Part model, mm, in its own coordinate system. Face numbers are marked on the shaded views. A direction names the side the tool comes from. Round coordinates to 2 decimals unless told otherwise and drop trailing zeros. Order: outer loops, then holes, each group sorted by start corner. A loop starts at its lowest first (then second) coordinate and runs counter-clockwise, first axis right, second up. Notation, with made-up numbers: (81.25, 75) - (112.25, 75) arc R18 ccw to (112.25, 88) - close; hole circle Ø1 at (-38.75, 68). An arc over 180 degrees is marked (long way). Return JSON: item names as keys, results as strings. Group by question number.
Item 1: Two-plate mould, pull along Z, no slides. Class the marked faces 3, 4, 5 and 6: released by +Z, released by -Z, zero draft, split by the parting line, or undercut.
Item 2: Drop flat-ended pins along their axis: pin 1 (10 mm diameter, centred on x = 39.878, z = -12.7, fed in from +Y) (3 decimals); pin 2 (0.5 mm diameter, centred on x = 24.5, z = -27, fed in from -Y); pin 3 (1.6 mm diameter, centred on x = 10.5, z = -27.5, fed in from -Y). Give the stop position or say it passes through.
Item 3: Tool access for the marked faces 1 and 2: list every direction of +Z, -Z, +X, -X, +Y, -Y with a clear straight run to the whole face (end or side of a thin tool).
Item 4: Probe probe 1 along Z at (x, y) = (29.5, 21) (3 decimals); probe 2 along Y at (x, z) = (12, -27); probe 3 along X at (y, z) = (30, -26). List the from-to ranges inside material, lowest first.
Item 5: Saw through at C-C on y = 30.48. List the corners of the cut face in (x, z) (3 decimals), and give its area (3 significant figures).
Item 6: Saw through at D-D on z = -15. List the corners of the cut face in (x, y) (3 decimals), and give its area (3 significant figures).
Item 7: Saw through at B-B on x = 18.5. List the corners of the cut face in (y, z) (3 decimals), and give its area (3 significant figures).
Item 8: Saw through at A-A on x = 12.7. State how many separate pieces and enclosed holes the cut face has, and give its area (3 significant figures).
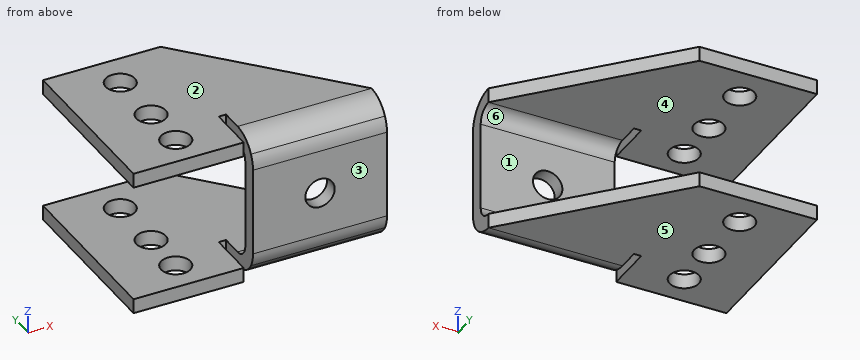
```python
from build123d import *

# Parameters (mm, degrees)
BOSS_EXTRUDE1_DEPTH     = 3.175
SKETCH2_W               = 28.956
SKETCH2_H               = 3.175
BOSS_EXTRUDE2_DEPTH     = 25.4
CUT_EXTRUDE1_DEPTH      = 74.581568589
CUT_EXTRUDE1_DEPTH_BACK = 74.581568589
SKETCH3_R               = 3.175
CUT_EXTRUDE2_DEPTH      = 71.646025975
CUT_EXTRUDE2_DEPTH_BACK = 71.646025975
SKETCH6_R               = 3.175
CUT_EXTRUDE3_DEPTH      = 74.581568589
CUT_EXTRUDE3_DEPTH_BACK = 74.581568589
SKETCH7_W               = 25.4
SKETCH7_H               = 0.79375
CONVERT_SOLID1_START    = 23.8125
CONVERT_SOLID1_DEPTH    = 30.5435
CONVERT_SOLID1_2_DEPTH  = 1.5875
CONVERT_SOLID1_START_2  = 25.4
CONVERT_SOLID1_3_DEPTH  = 28.956


# Read off the part's stored shape, not the designer's step: Convert-Solid1
with BuildPart() as part:
    # Sketch1 → Boss-Extrude1 (new body)
    with BuildSketch(Plane.XY):
        Polygon((54.356, 6.35), (25.4, 38.1), (0, 38.1), (0, 0), (54.356, 0), align=None)
    boss_extrude1 = extrude(amount=BOSS_EXTRUDE1_DEPTH)

    # Sketch2 → Boss-Extrude2 (add)
    with BuildSketch(Plane(origin=(0, 0, 0), x_dir=(-1, 0, 0), z_dir=(0, 0, -1))):
        with Locations((-39.878, 1.5875)):
            Rectangle(SKETCH2_W, SKETCH2_H)
    extrude(amount=BOSS_EXTRUDE2_DEPTH)

    # Mirror1: Boss-Extrude1 across plane
    add(boss_extrude1.mirror(Plane.XY.offset(-12.7)))

    # Sketch3 → Cut-Extrude1 (cut, two sides: drawn at the far end of the back side and taken through both)
    with BuildSketch(Plane.XY.offset(3.175).offset(-CUT_EXTRUDE1_DEPTH_BACK)):
        with Locations((12.7, 7.62)):
            Circle(SKETCH3_R)
        with Locations((12.7, 17.78)):
            Circle(SKETCH3_R)
        with Locations((12.7, 30.48)):
            Circle(SKETCH3_R)
    extrude(amount=CUT_EXTRUDE1_DEPTH + CUT_EXTRUDE1_DEPTH_BACK, mode=Mode.SUBTRACT)

    # Sketch6 → Cut-Extrude2 (cut, two sides: drawn at the far end of the back side and taken through both)
    with BuildSketch(Plane(origin=(0, 3.175, 0), x_dir=(1, 0, 0), z_dir=(0, 1, 0)).offset(-CUT_EXTRUDE2_DEPTH_BACK)):
        with Locations(Location((39.878, 12.7, 0), (0, 0, 270))):
            Circle(SKETCH6_R)
    extrude(amount=CUT_EXTRUDE2_DEPTH + CUT_EXTRUDE2_DEPTH_BACK, mode=Mode.SUBTRACT)

    # Sketch7 → Cut-Extrude3 (cut, two sides: drawn at the far end of the back side and taken through both)
    with BuildSketch(Plane(origin=(0, 0, -28.575), x_dir=(-1, 0, 0), z_dir=(0, 0, -1)).offset(-CUT_EXTRUDE3_DEPTH_BACK)):
        with Locations((-12.7, 0.396875)):
            Rectangle(SKETCH7_W, SKETCH7_H)
    extrude(amount=CUT_EXTRUDE3_DEPTH + CUT_EXTRUDE3_DEPTH_BACK, mode=Mode.SUBTRACT)

    # Convert-Solid1 outline → Convert-Solid1 (cut)
    with BuildSketch(Plane.YZ.offset(CONVERT_SOLID1_START)):
        with BuildLine():
            Line((0, -28.575), (6.35, -28.575))
            ThreePointArc((6.35, -28.575), (3.174999999, -27.724261314), (0.850738685, -25.4))
            ThreePointArc((0.850738685, -25.4), (0.216371003, -23.868500936), (0, -22.225))
            Line((0, -22.225), (0, -28.575))
        make_face()
        with BuildLine():
            Line((0, 3.175), (0, -3.175))
            ThreePointArc((0, -3.175), (0.216371003, -1.531499064), (0.850738685, 0))
            ThreePointArc((0.850738685, 0), (3.174999999, 2.324261314), (6.35, 3.175))
            Line((6.35, 3.175), (0, 3.175))
        make_face()
    extrude(amount=CONVERT_SOLID1_DEPTH, mode=Mode.SUBTRACT)

    # Convert-Solid1 2 outline → Convert-Solid1 2 (cut)
    with BuildSketch(Plane.YZ.offset(CONVERT_SOLID1_START)):
        with BuildLine():
            Line((6.35, -28.575), (11.1125, -28.575))
            Line((11.1125, -28.575), (11.1125, -25.4))
            Line((11.1125, -25.4), (0.850738685, -25.4))
            ThreePointArc((0.850738685, -25.4), (3.174999999, -27.724261314), (6.35, -28.575))
        make_face()
        with BuildLine():
            Line((0.850738685, 0), (11.1125, 0))
            Line((11.1125, 0), (11.1125, 3.175))
            Line((11.1125, 3.175), (6.35, 3.175))
            ThreePointArc((6.35, 3.175), (3.174999999, 2.324261314), (0.850738685, 0))
        make_face()
    extrude(amount=CONVERT_SOLID1_2_DEPTH, mode=Mode.SUBTRACT)

    # Convert-Solid1 3 outline → Convert-Solid1 3 (add)
    with BuildSketch(Plane.YZ.offset(CONVERT_SOLID1_START_2)):
        with BuildLine():
            Line((3.175, -25.4), (6.35, -25.4))
            ThreePointArc((6.35, -25.4), (4.10493597, -24.47006403), (3.175, -22.225))
            Line((3.175, -22.225), (3.175, -25.4))
        make_face()
        with BuildLine():
            Line((3.175, 0), (3.175, -3.175))
            ThreePointArc((3.175, -3.175), (4.10493597, -0.92993597), (6.35, 0))
            Line((6.35, 0), (3.175, 0))
        make_face()
    extrude(amount=CONVERT_SOLID1_3_DEPTH)


solid = part.part
```
Filled in:
{
 "1": {"face 3": "zero draft", "face 4": "undercut", "face 5": "released by -Z", "face 6": "undercut"},
 "2": {"pin 1": "stops at y = 3.175", "pin 2": "stops at y = 11.11", "pin 3": "stops at y = 0.79"},
 "3": {"face 1": "+X, -X, +Y", "face 2": "+Z, +X, -X, +Y, -Y"},
 "4": {"probe 1": "z = -28.575 to -25.4, 0 to 3.175", "probe 2": "y = 0.79 to 4.52, 10.72 to 14.68, 20.88 to 27.38, 33.58 to 38.1", "probe 3": "x = 0 to 9.56, 15.84 to 32.79"},
 "5": {"outline": "(0, -28.575) - (9.525, -28.575) - (9.525, -25.4) - (0, -25.4) - close; (0, 0) - (9.525, 0) - (9.525, 3.175) - (0, 3.175) - close; (15.875, -28.575) - (32.349, -28.575) - (32.349, -25.4) - (15.875, -25.4) - close; (15.875, 0) - (32.349, 0) - (32.349, 3.175) - (15.875, 3.175) - close", "area": "165 mm^2"},
 "6": {"outline": "(25.4, 0) - (37.689, 0) - (37.689, 3.175) - (25.4, 3.175) - close; (42.067, 0) - (54.356, 0) - (54.356, 3.175) - (42.067, 3.175) - close", "area": "78.0 mm^2"},
 "7": {"outline": "(0.794, -28.575) - (38.1, -28.575) - (38.1, -25.4) - (0.794, -25.4) - close; (0.794, 0) - (38.1, 0) - (38.1, 3.175) - (0.794, 3.175) - close", "area": "237 mm^2"},
 "8": {"separate pieces": "8", "enclosed holes": "0", "area": "116 mm^2"}
}
